Part model, mm, in its own coordinate system. A direction names the side the tool comes from. Give positions to 0.01 mm unless a question says otherwise; leave off trailing zeros. Loops run counter-clockwise (first coordinate to the right, second up) from the corner with the lowest first, then second, coordinate; pieces in that order, holes last. Notation, with made-up numbers: M 49.5,-39 L 71.5,-39 A19 ccw 71.5,-16 Z; hole C -14,-13 d5. An arc over 180 degrees is marked long. Answer in a Markdown table with one row per item.
from build123d import *
from build123d.topology import SkipClean

# Parameters (mm, degrees)
SKETCH1_W                   = 102
SKETCH1_H                   = 102
BOSS_EXTRUDE1_DEPTH         = 50
CUT_EXTRUDE_THIN1_OUTLINE_W = 40
CUT_EXTRUDE_THIN1_OUTLINE_H = 95.773670058
CUT_EXTRUDE_THIN1_DEPTH     = 50
SKETCH4_W                   = 40
SKETCH4_H                   = 6.202657501
CUT_EXTRUDE3_DEPTH          = 54
SKETCH5_W                   = 33.817621941
SKETCH5_H                   = 102.594578927
CUT_EXTRUDE4_DEPTH          = 20
SKETCH6_W                   = 27.820383201
SKETCH6_H                   = 98.886835029
CUT_EXTRUDE5_DEPTH          = 20
SKETCH7_W                   = 30.8
SKETCH7_H                   = 3.364819678
BOSS_EXTRUDE2_DEPTH         = 21
SKETCH9_W                   = 31
SKETCH9_H                   = 3.479961613
BOSS_EXTRUDE4_DEPTH         = 21
SKETCH11_W                  = 98.820383201
SKETCH11_H                  = 3.113164971
BOSS_EXTRUDE6_DEPTH         = 47.625
SKETCH14_W                  = 102
SKETCH14_H                  = 5
CUT_EXTRUDE7_DEPTH          = 105
SKETCH17_R                  = 7
CUT_EXTRUDE12_DEPTH         = 20.5
M3_CLEARANCE_HOLE1_D        = 3.4
SKETCH22_W                  = 3.179616799
SKETCH22_H                  = 102
BOSS_EXTRUDE7_DEPTH         = 47.6


# Read off the part's stored shape, not the designer's step: Cut-Extrude-Thin1
with BuildPart() as part:
    # Sketch1 → Boss-Extrude1 (new body)
    with BuildSketch(Plane(origin=(0, 0, 0), x_dir=(1, 0, 0), z_dir=(0, 1, 0))):
        with Locations((-66.567363259, 25.977216604)):
            Rectangle(SKETCH1_W, SKETCH1_H)
    extrude(amount=BOSS_EXTRUDE1_DEPTH)

    # Sketch2 → Cut-Revolve1 (revolve, cut)
    with SkipClean():  # the faces are left unmerged after this step: merging them gives an invalid solid
        with BuildSketch(Plane(origin=(0, 0, 0), x_dir=(1, 0, 0), z_dir=(0, 1, 0))):
            with BuildLine():
                ThreePointArc((-66.567363259, 73.602216604), (-114.192363259, 25.977216604), (-66.567363259, -21.647783396))
                Line((-66.567363259, -21.647783396), (-66.567363259, 73.602216604))
            make_face()
            with BuildLine():
                Line((-66.567363259, 73.602216604), (-66.567363259, -21.647783396))
                ThreePointArc((-66.567363259, -21.647783396), (-32.891402805, -7.69874385), (-18.942363259, 25.977216604))
                ThreePointArc((-18.942363259, 25.977216604), (-32.891402805, 59.653177058), (-66.567363259, 73.602216604))
            make_face()
        revolve(axis=Axis((-66.567363259, 0, 21.647783396), (0, 0, -1)), mode=Mode.SUBTRACT)
    add(part.part.scale(1), mode=Mode.REPLACE)  # the faces are merged on a copy

    # Cut-Extrude-Thin1 outline → Cut-Extrude-Thin1 (cut)
    with BuildSketch(Plane(origin=(0, 0, 0), x_dir=(1, 0, 0), z_dir=(0, 1, 0))):
        with Locations((-66.567363259, 25.977216604)):
            Rectangle(CUT_EXTRUDE_THIN1_OUTLINE_W, CUT_EXTRUDE_THIN1_OUTLINE_H)
    extrude(amount=CUT_EXTRUDE_THIN1_DEPTH, mode=Mode.SUBTRACT)

    # Sketch4 → Cut-Extrude3 (cut)
    with BuildSketch(Plane(origin=(0, 0, 0), x_dir=(1, 0, 0), z_dir=(0, 1, 0))):
        with Locations((-66.567363259, -25.010947176)):
            Rectangle(SKETCH4_W, SKETCH4_H)
    extrude(amount=CUT_EXTRUDE3_DEPTH, mode=Mode.SUBTRACT)

    # Sketch5 → Cut-Extrude4 (cut)
    with BuildSketch(Plane(origin=(0, 0, 0), x_dir=(1, 0, 0), z_dir=(0, 1, 0))):
        with Locations((-29.658552289, 22.56676217)):
            Rectangle(SKETCH5_W, SKETCH5_H)
    extrude(amount=CUT_EXTRUDE4_DEPTH, mode=Mode.SUBTRACT)

    # Sketch6 → Cut-Extrude5 (cut)
    with BuildSketch(Plane(origin=(0, 0, 0), x_dir=(-1, 0, 0), z_dir=(0, -1, 0))):
        with Locations((100.47755486, 24.420634119)):
            Rectangle(SKETCH6_W, SKETCH6_H)
    extrude(amount=-CUT_EXTRUDE5_DEPTH, mode=Mode.SUBTRACT)

    # Sketch7 → Boss-Extrude2 (add)
    with BuildSketch(Plane(origin=(0, 0, 0), x_dir=(1, 0, 0), z_dir=(0, 1, 0))):
        with Locations((-102.167363259, -23.340373557)):
            Rectangle(SKETCH7_W, SKETCH7_H)
    extrude(amount=BOSS_EXTRUDE2_DEPTH)

    # Sketch9 → Boss-Extrude4 (add)
    with BuildSketch(Plane.XZ.offset(-20)):
        with Locations((-31.067363259, 23.28280259)):
            Rectangle(SKETCH9_W, SKETCH9_H)
    extrude(amount=BOSS_EXTRUDE4_DEPTH)

    # Sketch11 → Boss-Extrude6 (add)
    with BuildSketch(Plane.XZ):
        with Locations((-64.97755486, -75.420634119)):
            Rectangle(SKETCH11_W, SKETCH11_H)
    extrude(amount=BOSS_EXTRUDE6_DEPTH)

    # Sketch14 → Cut-Extrude7 (cut)
    with BuildSketch(Plane(origin=(-15.567363259, 0, 0), x_dir=(0, 0, -1), z_dir=(1, 0, 0))):
        with Locations((25.977216604, 47.5)):
            Rectangle(SKETCH14_W, SKETCH14_H)
    extrude(amount=-CUT_EXTRUDE7_DEPTH, mode=Mode.SUBTRACT)

    # Sketch17 → Cut-Extrude12 (cut)
    with BuildSketch(Plane.XZ.offset(-20)):
        with Locations(Location((-94.167363259, 1.657963718, 0), (0, 0, 270))):
            Circle(SKETCH17_R)
        with Locations(Location((-94.167363259, -53.864051633, 0), (0, 0, 284.685382437))):
            Circle(SKETCH17_R)
        with Locations(Location((-39.167363259, 1.657963718, 0), (0, 0, 349.246729183))):
            Circle(SKETCH17_R)
        with Locations(Location((-39.167363259, -53.864051633, 0), (0, 0, 270))):
            Circle(SKETCH17_R)
    extrude(amount=-CUT_EXTRUDE12_DEPTH, mode=Mode.SUBTRACT)

    # M3 Clearance Hole1 (through all)
    with Locations(Plane(origin=(0, 40.5, 0), x_dir=(-1, 0, 0), z_dir=(0, -1, 0))):
        with Locations((94.167363259, -1.657963718), (39.167363259, -1.657963718), (39.167363259, 53.864051633), (94.167363259, 53.864051633)):
            Hole(M3_CLEARANCE_HOLE1_D / 2)

    # Sketch22 → Boss-Extrude7 (add)
    with BuildSketch(Plane.XZ):
        with Locations((-115.97755486, -25.977216604)):
            Rectangle(SKETCH22_W, SKETCH22_H)
    extrude(amount=BOSS_EXTRUDE7_DEPTH)


solid = part.part
(1) Saw through at A-A (y = 5). Write the cut outline in (x, z), plus the area to 3 significant figures.
Recorded:
| item | result |
|---|---|
| outline | M -117.57,-76.98 L -15.57,-76.98 L -15.57,-73.86 L -114.39,-73.86 L -114.39,21.66 L -86.77,21.66 L -86.77,25.02 L -117.57,25.02 Z; M -46.57,21.54 L -15.57,21.54 L -15.57,25.02 L -46.57,25.02 Z |
| area | 833 mm^2 |
(2) Saw through at B-B (z = -22.5). Write the cut outline in (x, y), plus the area to 3 significant figures.
Recorded:
| item | result |
|---|---|
| outline | M -117.57,-47.6 L -114.39,-47.6 L -114.39,20 L -109.65,20 A47.5 cw -86.57,43.08 L -86.57,45 L -117.57,45 Z; M -46.57,43.08 A47.5 cw -23.49,20 L -15.57,20 L -15.57,45 L -46.57,45 Z |
| area | 1,110 mm^2 |
(3) Pin check, flat tips, straight feed: pin 1 Ø3 at (y, z) = (-16.5, -33) entering from +X; pin 2 Ø1.5 at (x, z) = (-88, 14.5) entering from -Y; pin 3 Ø5 at (x, z) = (-104, -40.5) entering from -Y. Stop position of each tip, or through.
Recorded:
| item | result |
|---|---|
| pin 1 | stops at x = -114.39 |
| pin 2 | stops at y = 20 |
| pin 3 | stops at y = 21.19 |
(4) Pull direction X, two halves, no side cores. Call faces 1 (the face through (-98.43, 32.38, 7.21)), 2 (the face through (-117.567, -1, -27)), 3 (the face through (-102, 20, 25.023)), 4 (the face through (-86.567, 43.4, -23.7)): +X half, -X half, draft (parallel to the pull), parting line (faces both ways), or undercut.
Recorded:
| item | result |
|---|---|
| face 1 | undercut |
| face 2 | -X half |
| face 3 | draft |
| face 4 | undercut |
(5) Saw through at D-D (y = -26). Write the cut outline in (x, z).
Recorded:
| item | result |
|---|---|
| outline | M -117.57,-76.98 L -15.57,-76.98 L -15.57,-73.86 L -114.39,-73.86 L -114.39,25.02 L -117.57,25.02 Z |
(6) Saw through at C-C (y = 36). Write the cut outline in (x, z).
Recorded:
| item | result |
|---|---|
| outline | M -117.57,-76.98 L -15.57,-76.98 L -15.57,25.02 L -46.57,25.02 L -46.57,-2.06 A31.18 cw -46.57,-49.9 L -46.57,-73.86 L -86.57,-73.86 L -86.57,-49.9 A31.18 cw -86.57,-2.06 L -86.57,25.02 L -117.57,25.02 Z; hole C -94.17,-53.86 d14; hole C -94.17,1.66 d14; hole C -39.17,-53.86 d14; hole C -39.17,1.66 d14 |
(7) Which spindle directions (+Z, -Z, +X, -X, +Y, -Y) get a long thin tool onto all of the face, cutting with end or side? Do faces 5 (the face through (-99.36, 32.38, -58.56)), 6 (the face through (-31, 10, 21.543)), 7 (the face through (-43, 45, -25)), 8 (the face through (-46.567, 44, -21)). Say none if no direction does.
Recorded:
| item | result |
|---|---|
| face 5 | -Y |
| face 6 | +X, -Y |
| face 7 | +Z, -Z, +X, -X, +Y |
| face 8 | +Z, +Y, -Y |
(8) Drill centre lines: line 1 along X through (y, z) = (40, 1); line 2 along Z through (x, y) = (-103.5, 1); line 3 along Z through (x, y) = (-91.5, -20.5). Where is each one in solid material? Low to high.
Recorded:
| item | result |
|---|---|
| line 1 | x = -117.57 to -101.14, -87.2 to -86.57, -46.57 to -46.14, -32.2 to -15.57 |
| line 2 | z = -76.98 to -73.86, 21.66 to 25.02 |
| line 3 | z = -76.98 to -73.86 |
